```python
from build123d import *

# Parameters (mm, degrees)
SKETCH1_R           = 25
SKETCH1_R_2         = 15
BOSS_EXTRUDE1_DEPTH = 10
BOSS_EXTRUDE2_DEPTH = 5


with BuildPart() as part:
    # Sketch1 → Boss-Extrude1 (new, symmetric)
    # profile 1 of 6: a face of its own
    with BuildSketch(Plane(origin=(0, 0, 0), x_dir=(1, 0, 0), z_dir=(0, 1, 0))):
        Circle(SKETCH1_R)
        with Locations(Location((0, 0, 0), (0, 0, 270))):
            Circle(SKETCH1_R_2, mode=Mode.SUBTRACT)
    # profile 2 of 6: a face of its own
    with BuildSketch(Plane(origin=(0, 0, 0), x_dir=(1, 0, 0), z_dir=(0, 1, 0))):
        with BuildLine():
            ThreePointArc((-16.364080859, 18.900181419), (-11.349762493, 22.275163105), (-5.672002568, 24.348067415))
            Line((-5.672002568, 24.348067415), (-13.525991536, 39.762388673))
            ThreePointArc((-13.525991536, 39.762388673), (-19.067600989, 37.422274016), (-24.218069826, 34.314502676))
            Line((-24.218069826, 34.314502676), (-16.364080859, 18.900181419))
        make_face()
    # profile 3 of 6: a face of its own
    with BuildSketch(Plane(origin=(0, 0, 0), x_dir=(1, 0, 0), z_dir=(0, 1, 0))):
        with BuildLine():
            Line((-0.576728553, -41.996040101), (2.129571608, -24.90913336))
            ThreePointArc((2.129571608, -24.90913336), (-3.910861626, -24.692208515), (-9.722688479, -23.03191978))
            Line((-9.722688479, -23.03191978), (-12.42898864, -40.118826521))
            ThreePointArc((-12.42898864, -40.118826521), (-6.570247532, -41.482910305), (-0.576728553, -41.996040101))
        make_face()
    # profile 4 of 6: a face of its own
    with BuildSketch(Plane(origin=(0, 0, 0), x_dir=(1, 0, 0), z_dir=(0, 1, 0))):
        with BuildLine():
            ThreePointArc((-23.03191978, -9.722688479), (-24.692208515, -3.910861626), (-24.90913336, 2.129571608))
            Line((-24.90913336, 2.129571608), (-41.996040101, -0.576728553))
            ThreePointArc((-41.996040101, -0.576728553), (-41.482910305, -6.570247532), (-40.118826521, -12.42898864))
            Line((-40.118826521, -12.42898864), (-23.03191978, -9.722688479))
        make_face()
    # profile 5 of 6: a face of its own
    with BuildSketch(Plane(origin=(0, 0, 0), x_dir=(1, 0, 0), z_dir=(0, 1, 0))):
        with BuildLine():
            ThreePointArc((12.918361615, 21.403642989), (17.67766953, 17.67766953), (21.403642989, 12.918361615))
            Line((21.403642989, 12.918361615), (33.636517601, 25.151236226))
            ThreePointArc((33.636517601, 25.151236226), (29.69848481, 29.69848481), (25.151236226, 33.636517601))
            Line((25.151236226, 33.636517601), (12.918361615, 21.403642989))
        make_face()
    # profile 6 of 6: a face of its own
    with BuildSketch(Plane(origin=(0, 0, 0), x_dir=(1, 0, 0), z_dir=(0, 1, 0))):
        with BuildLine():
            Line((39.762388673, -13.525991536), (24.348067415, -5.672002568))
            ThreePointArc((24.348067415, -5.672002568), (22.275163105, -11.349762493), (18.900181419, -16.364080859))
            Line((18.900181419, -16.364080859), (34.314502676, -24.218069826))
            ThreePointArc((34.314502676, -24.218069826), (37.422274016, -19.067600989), (39.762388673, -13.525991536))
        make_face()
    extrude(amount=BOSS_EXTRUDE1_DEPTH, both=True)

    # Sketch1_3 → Boss-Extrude2 (add, symmetric)
    with BuildSketch(Plane(origin=(0, 0, 0), x_dir=(1, 0, 0), z_dir=(0, 1, 0))):
        with BuildLine():
            Line((57, -17.916472867), (57, -30))
            ThreePointArc((57, -30), (72, -45), (87, -30))
            Line((87, -30), (87, 30))
            ThreePointArc((87, 30), (72, 45), (57, 30))
            Line((57, 30), (57, 17.916472867))
            ThreePointArc((57, 17.916472867), (52.825722824, 12.985126011), (47.272727273, 16.287702607))
            ThreePointArc((47.272727273, 16.287702607), (0, 50), (-47.272727273, 16.287702607))
            ThreePointArc((-47.272727273, 16.287702607), (-52.825722824, 12.985126011), (-57, 17.916472867))
            Line((-57, 17.916472867), (-57, 30))
            ThreePointArc((-57, 30), (-72, 45), (-87, 30))
            Line((-87, 30), (-87, -30))
            ThreePointArc((-87, -30), (-72, -45), (-57, -30))
            Line((-57, -30), (-57, -17.916472867))
            ThreePointArc((-57, -17.916472867), (-52.825722824, -12.985126011), (-47.272727273, -16.287702607))
            ThreePointArc((-47.272727273, -16.287702607), (0, -50), (47.272727273, -16.287702607))
            ThreePointArc((47.272727273, -16.287702607), (52.825722824, -12.985126011), (57, -17.916472867))
        make_face()
        with BuildLine():
            Line((-82, -30), (-82, 30))
            ThreePointArc((-82, 30), (-72, 40), (-62, 30))
            Line((-62, 30), (-62, -30))
            ThreePointArc((-62, -30), (-72, -40), (-82, -30))
        make_face(mode=Mode.SUBTRACT)
        with BuildLine():
            Line((33.636517601, 25.151236226), (21.403642989, 12.918361615))
            ThreePointArc((21.403642989, 12.918361615), (24.084134557, 6.704808919), (25, 0))
            ThreePointArc((25, 0), (24.836482092, -2.85467289), (24.348067415, -5.672002568))
            Line((24.348067415, -5.672002568), (39.762388673, -13.525991536))
            ThreePointArc((39.762388673, -13.525991536), (37.422274016, -19.067600989), (34.314502676, -24.218069826))
            Line((34.314502676, -24.218069826), (18.900181419, -16.364080859))
            ThreePointArc((18.900181419, -16.364080859), (11.349762493, -22.275163105), (2.129571608, -24.90913336))
            Line((2.129571608, -24.90913336), (-0.576728553, -41.996040101))
            ThreePointArc((-0.576728553, -41.996040101), (-6.570247532, -41.482910305), (-12.42898864, -40.118826521))
            Line((-12.42898864, -40.118826521), (-9.722688479, -23.03191978))
            ThreePointArc((-9.722688479, -23.03191978), (-17.67766953, -17.67766953), (-23.03191978, -9.722688479))
            Line((-23.03191978, -9.722688479), (-40.118826521, -12.42898864))
            ThreePointArc((-40.118826521, -12.42898864), (-41.482910305, -6.570247532), (-41.996040101, -0.576728553))
            Line((-41.996040101, -0.576728553), (-24.90913336, 2.129571608))
            ThreePointArc((-24.90913336, 2.129571608), (-22.275163105, 11.349762493), (-16.364080859, 18.900181419))
            Line((-16.364080859, 18.900181419), (-24.218069826, 34.314502676))
            ThreePointArc((-24.218069826, 34.314502676), (-19.067600989, 37.422274016), (-13.525991536, 39.762388673))
            Line((-13.525991536, 39.762388673), (-5.672002568, 24.348067415))
            ThreePointArc((-5.672002568, 24.348067415), (3.910861626, 24.692208515), (12.918361615, 21.403642989))
            Line((12.918361615, 21.403642989), (25.151236226, 33.636517601))
            ThreePointArc((25.151236226, 33.636517601), (29.69848481, 29.69848481), (33.636517601, 25.151236226))
        make_face(mode=Mode.SUBTRACT)
        with BuildLine():
            ThreePointArc((62, 30), (72, 40), (82, 30))
            Line((82, 30), (82, -30))
            ThreePointArc((82, -30), (72, -40), (62, -30))
            Line((62, -30), (62, 30))
        make_face(mode=Mode.SUBTRACT)
    extrude(amount=BOSS_EXTRUDE2_DEPTH, both=True)


solid = part.part
```
The model under review builds one solid part; all positions refer to its coordinate system, in mm. A direction names the side the tool comes from. Give positions to 0.01 mm unless a question says otherwise; leave off trailing zeros. Write each loop counter-clockwise with the first axis right and the second up, starting at its lowest first coordinate (ties: lowest second). Pieces come first, ordered by that corner, then holes.
(1) For P1, Ø2, axis at x = -61, y = -5.5, coming from the +Z side; P2, Ø6, axis at x = -35, y = -1.5, coming from the +Z side; P3, Ø3, axis at x = -38, z = -27.5, coming from the -Y side, all flat-tipped, find the tip position at first contact; note any pin that passes through.
(2) To check wall thickness, follow L1, parallel to X at y = -1, z = 0; L2, parallel to X at y = -3.5, z = -37.5; L3, parallel to X at y = 2.25, z = 31.5. State the ranges of each line that lie inside material, in increasing order.
(3) Tool access review of faces 4 (the cylindrical face through (-72, 0, -40)), 5 (the flat face through (57, 0, -24)), 6 (the flat face through (32.163, 7.535, 9.654)), 7 (the cylindrical face through (11.229, 7.535, 22.336)), 8 (the cylindrical face through (-41.496, -7.465, 6.487)): name each direction out of +Z, -Z, +X, -X, +Y, -Y from which nothing blocks a thin tool from reaching the whole face with its end or side.
(4) The part is to be moulded in two halves that separate along Z. For faces 1 (the flat face through (-11.057, 7.465, 31.456)), 2 (the cylindrical face through (52.9, 0.1, -13)), 3 (the cylindrical face through (37.384, -7.465, 19.143)), say which applies: released by +Z, released by -Z, zero draft, split by the parting line, or undercut.
(5) Consider section A-A, the plane x = -72. Give the boundary of the cut face in (y, z).
(6) Consider section D-D, the plane x = 30. Give the boundary of the cut face in (y, z).
(7) Consider section B-B, the plane y = -0.5. Give the boundary of the cut face in (x, z).
(8) Consider section C-C, the plane z = -37. Give the boundary of the cut face in (x, y), and give its area (3 significant figures).
Returned:
1. P1: stops at z = 41.06
1. P2: stops at z = 38.42
1. P3: stops at y = -5
2. L1: x = -87 to -82, -62 to -15, 15 to 62, 82 to 87
2. L2: x = -84.99 to -78.61, -65.39 to -59.01, -33.07 to 33.07, 59.01 to 65.39, 78.61 to 84.99
2. L3: x = -86.92 to -81.89, -62.11 to -57.08, -38.83 to 38.83, 57.08 to 62.11, 81.89 to 86.92
3. face 4: +Y, -Y
3. face 5: -Z, +Y, -Y
3. face 6: +X, +Y
3. face 7: +Z, +Y
3. face 8: +Z, -X, -Y
4. face 1: undercut
4. face 2: released by -Z
4. face 3: released by +Z
5. outline: (-5, -45) - (5, -45) - (5, -40) - (-5, -40) - close; (-5, 40) - (5, 40) - (5, 45) - (-5, 45) - close
6. outline: (-10, -29.39) - (-5, -29.39) - (-5, -40) - (5, -40) - (5, -29.39) - (10, -29.39) - (10, -21.51) - (5, -21.51) - (5, 8.55) - (10, 8.55) - (10, 22.02) - (5, 22.02) - (5, 40) - (-5, 40) - (-5, 22.02) - (-10, 22.02) - (-10, 8.55) - (-5, 8.55) - (-5, -21.51) - (-10, -21.51) - close
7. outline: (-87, -30) arc R15 ccw to (-57, -30) - (-57, -17.92) arc R5 cw to (-47.27, -16.29) arc R50 ccw to (47.27, -16.29) arc R5 cw to (57, -17.92) - (57, -30) arc R15 ccw to (87, -30) - (87, 30) arc R15 ccw to (57, 30) - (57, 17.92) arc R5 cw to (47.27, 16.29) arc R50 ccw to (-47.27, 16.29) arc R5 cw to (-57, 17.92) - (-57, 30) arc R15 ccw to (-87, 30) - close; hole (-82, -30) arc R10 ccw to (-62, -30) - (-62, 30) arc R10 ccw to (-82, 30) - close; hole circle Ø30 at (0, 0); hole (62, -30) arc R10 ccw to (82, -30) - (82, 30) arc R10 ccw to (62, 30) - close
8. outline: (-85.27, -5) - (-79.14, -5) - (-79.14, 5) - (-85.27, 5) - close; (-64.86, -5) - (-58.73, -5) - (-58.73, 5) - (-64.86, 5) - close; (-33.63, -5) - (-19.87, -5) - (-19.87, -10) - (-12.12, -10) - (-12.12, -5) - (33.63, -5) - (33.63, 5) - (-12.12, 5) - (-12.12, 10) - (-19.87, 10) - (-19.87, 5) - (-33.63, 5) - close; (58.73, -5) - (64.86, -5) - (64.86, 5) - (58.73, 5) - close; (79.14, -5) - (85.27, -5) - (85.27, 5) - (79.14, 5) - close
8. area: 995 mm2
